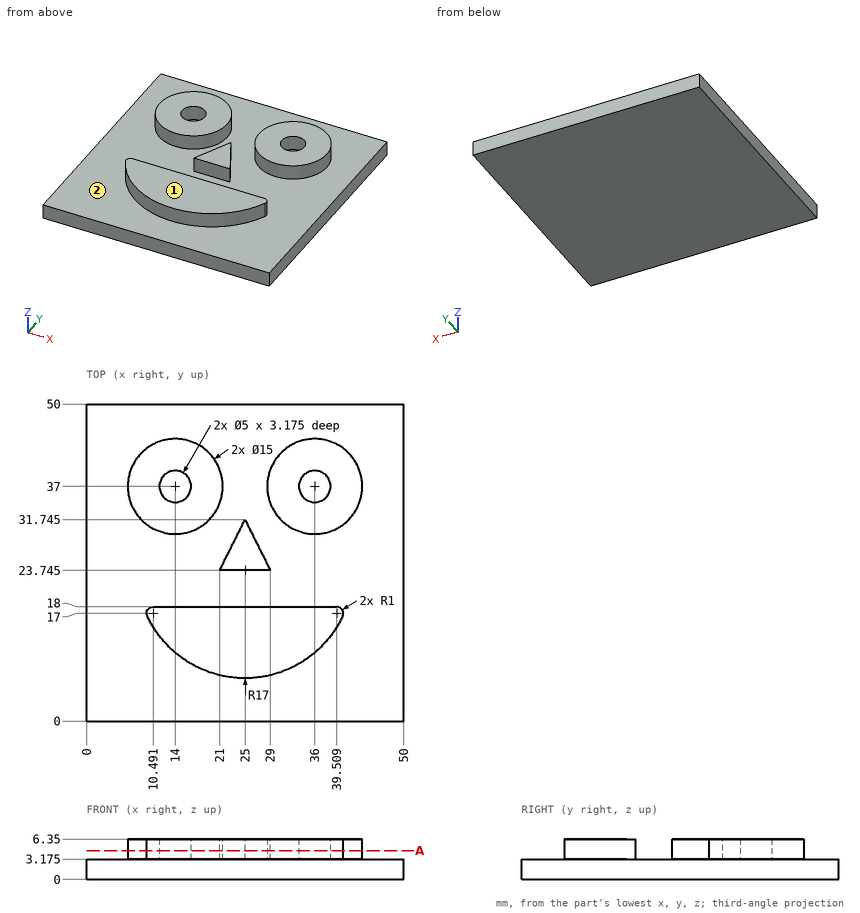
Drawing for the job (mm, zero at the part's lowest x, y, z). Give positions to 0.01 mm unless a question says otherwise; leave off trailing zeros. Order: outer loops, then holes, each group sorted by start corner. A loop starts at its lowest first (then second) coordinate and runs counter-clockwise, first axis right, second up. Notation, with made-up numbers: M -10.75,-34.5 L 28.25,-34.5 A27 cw 28.25,-18.5 Z; hole C 65,-23.75 d1. An arc over 180 degrees is marked long. Use a Markdown table: item, result. Add a question column.
(1) Saw through at A-A, the plane z = 4.5. Give the cut face in (x, y) (1 decimal).
(2) Mould opens along Y. For the marked faces 1 and 2 say: +Y half, -Y half, draft (parallel to the pull), parting line (faces both ways), or undercut.
(3) Probe line 1 along X through (y, z) = (35.5, 4.75); line 2 along Y through (x, z) = (36, 4.5) (1 decimal); line 3 along Z through (x, y) = (8.5, 12) (1 decimal). List the from-to ranges inside material, lowest first. Write a range as [from, to].
(4) Drop flat-ended pins along their axis: P1, Ø3.5, axis at x = 24.5, z = 5, coming from the +Y side (1 decimal); P2, Ø3, axis at x = 14, y = 37, coming from the +Z side (3 decimals). Give the stop position or say it passes through.
Answer key:
| question | item | result |
|---|---|---|
| 1 | outline | C 14,37 d15; M 9.6,16.6 A17 ccw 40.4,16.6 A1 ccw 39.5,18 L 10.5,18 A1 ccw Z; M 21,23.7 L 29,23.7 L 25,31.7 Z; C 36,37 d15; hole C 14,37 d5; hole C 36,37 d5 |
| 2 | face 1 | draft |
| 2 | face 2 | undercut |
| 3 | line 1 | [6.65, 12], [16, 21.35], [28.65, 34], [38, 43.35] |
| 3 | line 2 | [10.8, 18], [29.5, 34.5], [39.5, 44.5] |
| 3 | line 3 | [0, 3.2] |
| 4 | P1 | y = 31.7 |
| 4 | P2 | z = 3.175 |
